Geometry: final body of the model. Coordinates: model frame, mm. A direction names the side the tool comes from. Give positions to 0.01 mm unless a question says otherwise; leave off trailing zeros. Order: outer loops, then holes, each group sorted by start corner. A loop starts at its lowest first (then second) coordinate and runs counter-clockwise, first axis right, second up. Notation, with made-up numbers: (62, 87.25) -> (107, 87.25) arc R20 cw to (107, 97.25) -> close; hole circle Ø3 at (25.25, 11.25). An arc over 180 degrees is marked (long way). Answer in a Markdown table with one row per item. Add a question column.
Q1. Cut plane C-C on x = 8.5. Return the cut outline in (y, z), and give its area (3 significant figures).
Q2. Set-up query: faces 1 (the face through (5.2, 9.985, 16.2)), 2 (the face through (-5.7, 9.985, 16.5)), 3 (the face through (0, 5, -20)), 4 (the face through (0, 5, 20)), 5 (the face through (4.4, 9.985, 19.8)). Return all of +Z, -Z, +X, -X, +Y, -Y with unobstructed straight access to the full face (end or side cutting, diameter ignored); none if empty.
Q3. Line query: line 1 along X through (y, z) = (5.75, 0); line 2 along Z through (x, y) = (-9, 6.5); line 3 along Z through (x, y) = (4, 2.25). Output: solid intervals per line, ascending. Write a range as from..to.
Q4. Cut plane B-B on z = -5. Return the cut outline in (x, y), and give its area (3 significant figures).
Q5. Cut plane D-D on x = -2. Return the cut outline in (y, z) (3 decimals).
Q6. Cut plane A-A on y = 9. Return the cut outline in (x, z).
Q7. Contact query for flat-ended pins moving along their axis: P1, Ø2, axis at y = 5.5, z = 3.5, coming from the -X side; P2, Ø2, axis at x = -8.5, z = -5.5, coming from the +Y side; P3, Ø4, axis at x = 0.5, z = -10.5, coming from the +Y side; P4, Ø6, axis at y = 9.5, z = -15, coming from the -X side. Output: stop coordinate, or through.
from build123d import *

# Parameters (mm, degrees)
SKETCH1_R           = 12
BOSS_EXTRUDE1_DEPTH = 10
BOSS_EXTRUDE2_DEPTH = 5
BOSS_EXTRUDE3_DEPTH = 5


with BuildPart() as part:
    # Sketch1 → Boss-Extrude1 (new body)
    with BuildSketch(Plane(origin=(0, 0, 0), x_dir=(1, 0, 0), z_dir=(0, 1, 0))):
        with BuildLine():
            Line((-5.938922448, 19.097884704), (-4.65723572, 15.077087101))
            ThreePointArc((-4.65723572, 15.077087101), (-16.000205846, 0.123004291), (-4.888486885, -15.003702742))
            Line((-4.888486885, -15.003702742), (-6.195800868, -19.0160998))
            ThreePointArc((-6.195800868, -19.0160998), (-0.182924717, -19.999163446), (5.846927348, -19.12625004))
            Line((5.846927348, -19.12625004), (4.613225677, -15.090611282))
            ThreePointArc((4.613225677, -15.090611282), (15.53596231, -0.206998546), (4.736250871, 14.766121919))
            Line((4.736250871, 14.766121919), (6.108489826, 19.04432598))
            ThreePointArc((6.108489826, 19.04432598), (0.088912362, 19.999802364), (-5.938922448, 19.097884704))
        make_face()
        with Locations(Location((0, 0, 0), (0, 0, 270))):
            Circle(SKETCH1_R, mode=Mode.SUBTRACT)
    extrude(amount=BOSS_EXTRUDE1_DEPTH)

    # Sketch2 → Boss-Extrude2 (add)
    with BuildSketch(Plane(origin=(-0.182924717, 10, 19.999163446), x_dir=(0.9999581723101434, 0, 0.009146235846386387), z_dir=(-0.009146235846386385, 0, 0.9999581723101433))):
        Polygon((-5.97117687, -0.015009165), (5.99330158, -0.015009165), (-5.97117687, 2.885349138), align=None)
    extrude(amount=-BOSS_EXTRUDE2_DEPTH)

    # Sketch3 → Boss-Extrude3 (add)
    with BuildSketch(Plane(origin=(0.088912362, 10, -19.999802364), x_dir=(-0.9999901181910447, 0, -0.004445618096607563), z_dir=(0.004445618096607563, 0, -0.9999901181910447))):
        Polygon((-6.073960735, -0.007479705), (6.036027913, -0.007479705), (-6.073960735, 2.600191919), align=None)
    extrude(amount=-BOSS_EXTRUDE3_DEPTH)


solid = part.part
Completed:
| question | item | result |
|---|---|---|
| 1 | outline | (0, -12.95) -> (10, -12.95) -> (10, -8.47) -> (0, -8.47) -> close; (0, 8.47) -> (10, 8.47) -> (10, 13.23) -> (0, 13.23) -> close |
| 1 | area | 92.3 mm² |
| 2 | face 1 | +X, -Y |
| 2 | face 2 | -X, -Y |
| 2 | face 3 | -Z, -Y |
| 2 | face 4 | +Z, -Y |
| 2 | face 5 | +Z, +X, -Y |
| 3 | line 1 | x = -16..-12, 12..15.54 |
| 3 | line 2 | z = -13.07..-7.94, 7.94..13.06 |
| 3 | line 3 | z = -19.6..-11.31, 11.31..19.6 |
| 4 | outline | (-15.18, 0) -> (-10.91, 0) -> (-10.91, 10) -> (-15.18, 10) -> close; (10.91, 0) -> (14.67, 0) -> (14.67, 10) -> (10.91, 10) -> close |
| 4 | area | 80.4 mm² |
| 5 | outline | (0, -19.9) -> (9.993, -19.9) -> (9.993, -20.009) -> (10.842, -20.009) -> (10.847, -15.009) -> (10, -15.009) -> (10, -11.832) -> (0, -11.832) -> close; (0, 11.832) -> (10, 11.832) -> (10, 14.982) -> (11.889, 14.982) -> (11.878, 19.983) -> (9.985, 19.983) -> (9.985, 19.9) -> (0, 19.9) -> close |
| 6 | outline | (-6.2, 19.02) -> (-4.89, 15) arc R15.69 ccw to (-4.66, -15.08) -> (-5.94, -19.1) arc R20 ccw to (6.11, -19.04) -> (4.74, -14.77) arc R15.69 ccw to (4.61, 15.09) -> (5.85, 19.13) arc R20 ccw to start; hole circle Ø24 at (0, 0) |
| 7 | P1 | stops at x = -15.8 |
| 7 | P2 | passes through |
| 7 | P3 | stops at y = 10 |
| 7 | P4 | stops at x = -10.42 |
